Verification items for this drawing (mm, ordinates from the low corner). Give positions to 0.01 mm unless a question says otherwise; leave off trailing zeros. Order: outer loops, then holes, each group sorted by start corner. A loop starts at its lowest first (then second) coordinate and runs counter-clockwise, first axis right, second up. Notation, with made-up numbers: (11, -23) -> (66, -23) arc R16 ccw to (66, -18) -> close; hole circle Ø4 at (70.5, 12). An arc over 180 degrees is marked (long way). One line per question, with ' | ' between items.
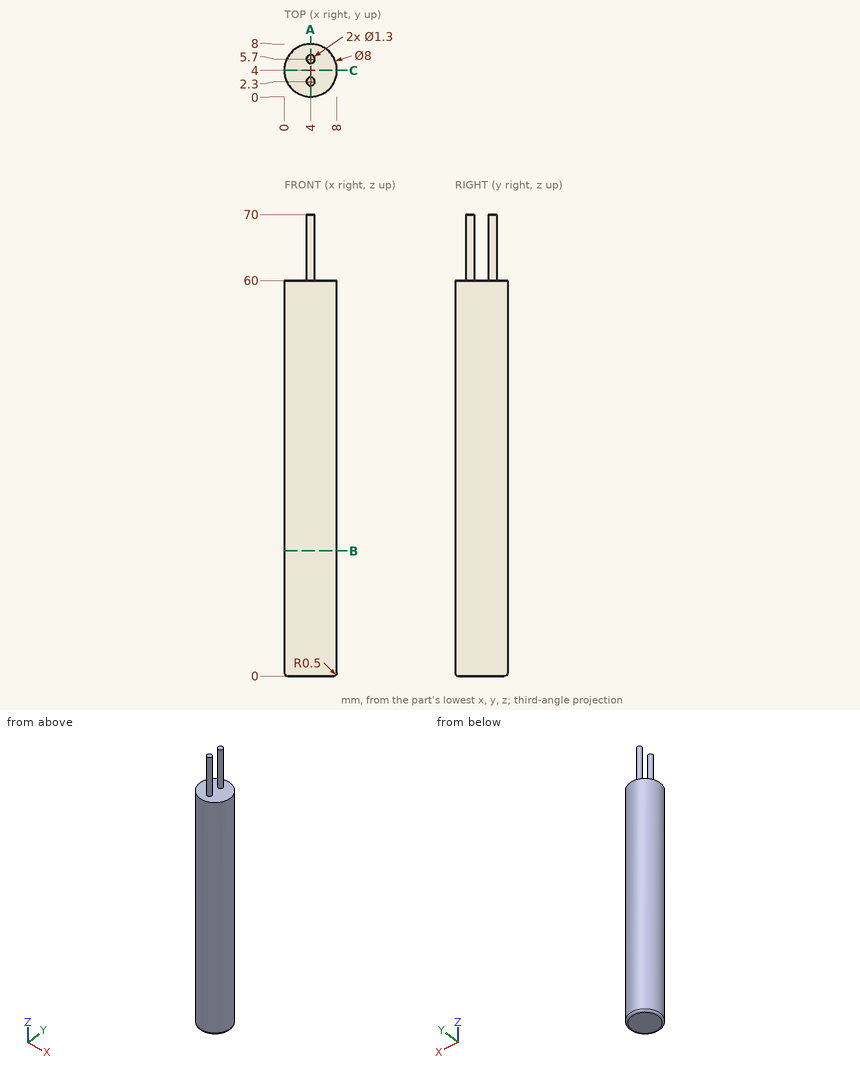
Q1. Section check A-A (x = 4). Enter the section's corners in (y, z).
Result sheet:
outline: (0, 0.5) arc R0.5 ccw to (0.5, 0) -> (7.5, 0) arc R0.5 ccw to (8, 0.5) -> (8, 60) -> (6.35, 60) -> (6.35, 70) -> (5.05, 70) -> (5.05, 60) -> (2.95, 60) -> (2.95, 70) -> (1.65, 70) -> (1.65, 60) -> (0, 60) -> close
Q2. Section check C-C (y = 4). Enter the section's corners in (x, z).
Result sheet:
outline: (0, 0.5) arc R0.5 ccw to (0.5, 0) -> (7.5, 0) arc R0.5 ccw to (8, 0.5) -> (8, 60) -> (0, 60) -> close
Q3. Thickness scan on line 1 (Y direction, x = 3.75, z = 28.5); line 2 (Y direction, x = 4.5, z = 66); line 3 (Z direction, x = 2.5, y = 7.25). Record the ranges inside material, lowest first.
Result sheet:
line 1: y = 0.01 to 7.99 | line 2: y = 1.88 to 2.72, 5.28 to 6.12 | line 3: z = 0.01 to 60
Q4. Depth check by flat-ended pin: pin 1 Ø4 at (y, z) = (1.5, 54) entering from -X; pin 2 Ø1.5 at (y, z) = (5.5, 31) entering from -X; pin 3 Ø3 at (y, z) = (1, 53) entering from -X. Enter the tip coordinate at first touch or a pass-through.
Result sheet:
pin 1: stops at x = 0.03 | pin 2: stops at x = 0.07 | pin 3: stops at x = 0.29
Q5. Section check B-B (z = 19). Enter the section's corners in (x, y).
Result sheet:
outline: circle Ø8 at (4, 4)
